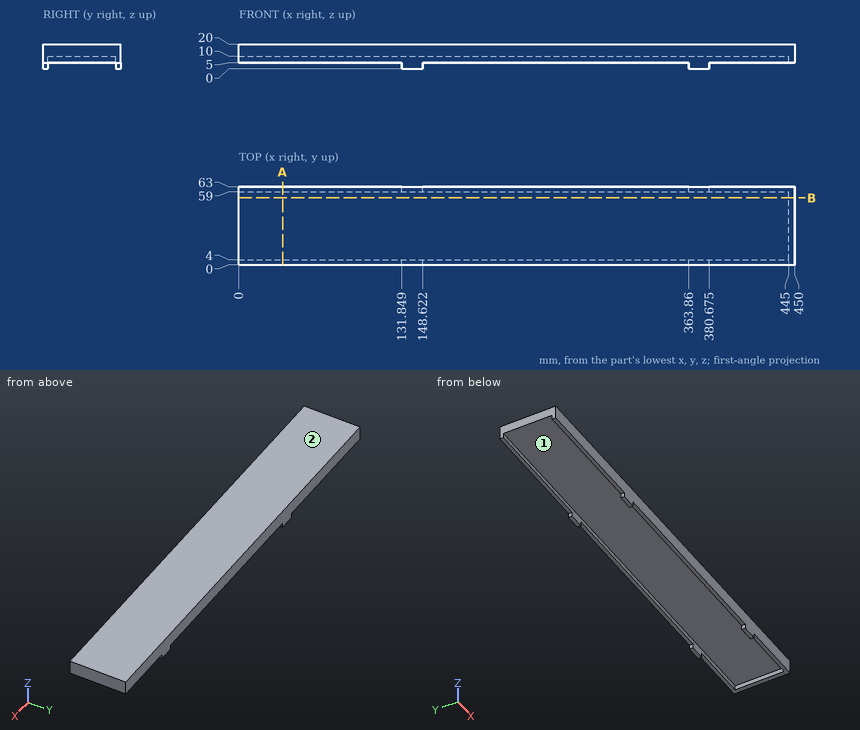
The drawing under review shows one solid part. Ordinate dimensions are in mm from its lowest x, y, z. Round coordinates to 2 decimals unless told otherwise and drop trailing zeros. Loops run counter-clockwise (first coordinate to the right, second up) from the corner with the lowest first, then second, coordinate; pieces in that order, holes last. Notation, with made-up numbers: (-14, 7) - (0, 7) arc R9 ccw to (0, 24) - close; hole circle Ø7 at (13, 34). An arc over 180 degrees is marked (long way). One line per item, written item: value. Start each with the question number.
1) Consider section B-B on y = 54. Give the boundary of the cut face in (x, z).
2) Insertion check: pin 1 Ø3 at (x, y) = (236.5, 3) entering from -Z; pin 2 Ø3 at (y, z) = (1.5, 3) entering from +X (1 decimal); pin 3 Ø3 at (y, z) = (2.5, 2.5) entering from -X. Each pin has a flat end and moves straight along its axis. Give the tip position at first contact, or say it passes through.
3) Draft analysis for pull direction Y (two halves, no side actions). For the marked faces 1 and 2, state which applies: +Y half, -Y half, draft (parallel to the pull), parting line (faces both ways), or undercut.
4) To check wall thickness, follow L1, parallel to Y at x = 222, z = 6.75; L2, parallel to X at y = 25, z = 7; L3, parallel to Z at x = 394, y = 43. State the ranges of each line that lie inside material, in increasing order. Write a range as from..to.
5) Consider section A-A on x = 35.5. Give the boundary of the cut face in (y, z), then the cut area to 3 significant figures.
Reported:
1. outline: (0, 10) - (445, 10) - (445, 5) - (450, 5) - (450, 20) - (0, 20) - close
2. pin 1: stops at z = 5
2. pin 2: stops at x = 380.7
2. pin 3: stops at x = 131.85
3. face 1: undercut
3. face 2: draft
4. L1: y = 0..4, 59..63
4. L2: x = 445..450
4. L3: z = 10..20
5. outline: (0, 5) - (4, 5) - (4, 10) - (59, 10) - (59, 5) - (63, 5) - (63, 20) - (0, 20) - close
5. area: 670 mm^2
